Build history of the part. All positions in model axes, mm. Face numbers are marked on the shaded views. A direction names the side the tool comes from. Round coordinates to 2 decimals unless told otherwise and drop trailing zeros. Write each loop counter-clockwise with the first axis right and the second up, starting at its lowest first coordinate (ties: lowest second). Pieces come first, ordered by that corner, then holes. Notation, with made-up numbers: (-35.5, -30) - (7.5, -30) arc R28 ccw to (7.5, -5) - close; hole circle Ø11 at (13, -22). An arc over 180 degrees is marked (long way). One line per question, with ' | ' between items.
from build123d import *

# Parameters (mm, degrees)
F0_W     = 11
F0_H     = 30
F1_DEPTH = 22
F3_DEPTH = 25
F4_R     = 5
F5_DEPTH = 11


with BuildPart() as f1:
    # F0 (on Right) → F1 (new body, symmetric)
    with BuildSketch(Plane.YZ):
        with BuildLine():
            Line((-56, 0), (-30, 0))
            ThreePointArc((-30, 0), (-29.4730143031, 5.5983415304), (-27.9105714739, 11))
            Line((-27.9105714739, 11), (-56, 11))
            Line((-56, 11), (-56, 0))
        make_face()
        with BuildLine():
            ThreePointArc((-27.9105714739, 11), (-29.4730143031, 5.5983415304), (-30, 0))
            Line((-30, 0), (-19, 0))
            ThreePointArc((-19, 0), (-18.1017503893, 5.7729223833), (-15.4919333848, 11))
            Line((-15.4919333848, 11), (-27.9105714739, 11))
        make_face()
        with BuildLine():
            Line((15.4919333848, 11), (27.9105714739, 11))
            ThreePointArc((27.9105714739, 11), (0, 30), (-27.9105714739, 11))
            Line((-27.9105714739, 11), (-15.4919333848, 11))
            ThreePointArc((-15.4919333848, 11), (0, 19), (15.4919333848, 11))
        make_face()
        with BuildLine():
            Line((19, 0), (30, 0))
            ThreePointArc((30, 0), (29.4730143031, 5.5983415304), (27.9105714739, 11))
            Line((27.9105714739, 11), (15.4919333848, 11))
            ThreePointArc((15.4919333848, 11), (18.1017503893, 5.7729223833), (19, 0))
        make_face()
        with BuildLine():
            ThreePointArc((27.9105714739, 11), (29.4730143031, 5.5983415304), (30, 0))
            Line((30, 0), (51, 0))
            Line((51, 0), (51, 11))
            Line((51, 11), (40, 11))
            Line((40, 11), (27.9105714739, 11))
        make_face()
        with Locations((45.5, 26)):
            Rectangle(F0_W, F0_H)
    extrude(amount=F1_DEPTH, both=True)

    # F2 (on face) → F3 (cut)
    with BuildSketch(Plane(origin=(0, 51, 0), x_dir=(-1, 0, 0), z_dir=(0, 1, 0))):
        with BuildLine():
            ThreePointArc((-6.5, 25), (0, 31.5), (6.5, 25))
            Line((6.5, 25), (6.5, 41))
            Line((6.5, 41), (-6.5, 41))
            Line((-6.5, 41), (-6.5, 25))
        make_face()
        with BuildLine():
            Line((-6.5, 25), (6.5, 25))
            ThreePointArc((6.5, 25), (0, 31.5), (-6.5, 25))
        make_face()
        with BuildLine():
            ThreePointArc((-6.5, 25), (0, 18.5), (6.5, 25))
            Line((6.5, 25), (-6.5, 25))
        make_face()
    extrude(amount=-F3_DEPTH, mode=Mode.SUBTRACT)

    # F4 (on face) → F5 (cut, through all)
    with BuildSketch(Plane.XY.offset(11)):
        with Locations((-11, -41.955285737)):
            Circle(F4_R)
        with Locations((11, -41.955285737)):
            Circle(F4_R)
    extrude(amount=-F5_DEPTH, mode=Mode.SUBTRACT)


solid = f1.part
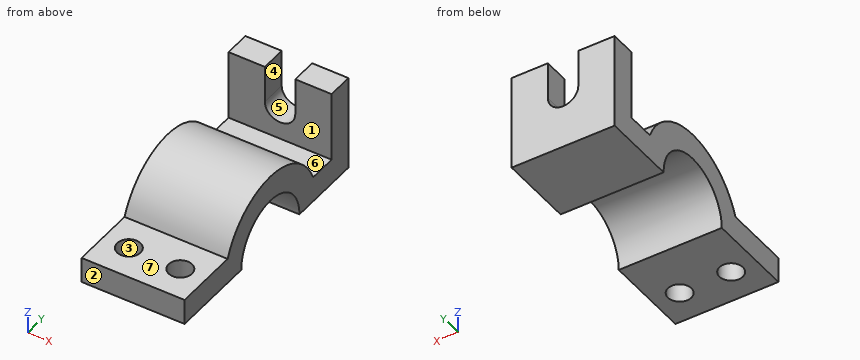
Q1. Saw through at A-A, the plane x = -11. List the corners of the cut face in (y, z).
Found:
outline: (-56, 0) - (-46.96, 0) - (-46.96, 11) - (-56, 11) - close; (-36.96, 0) - (-19, 0) arc R19 cw to (19, 0) - (51, 0) - (51, 41) - (40, 41) - (40, 11) - (27.91, 11) arc R30 ccw to (-27.91, 11) - (-36.96, 11) - close
Q2. Saw through at B-B, the plane z = 13.5. List the corners of the cut face in (x, y), then the cut area to 3 significant figures.
Found:
outline: (-22, -26.79) - (22, -26.79) - (22, -13.37) - (-22, -13.37) - close; (-22, 13.37) - (22, 13.37) - (22, 26.79) - (-22, 26.79) - close; (-22, 40) - (22, 40) - (22, 51) - (-22, 51) - close | area: 1,670 mm^2
Q3. Saw through at D-D, the plane x = 2.5. List the corners of the cut face in (y, z), then the cut area to 3 significant figures.
Found:
outline: (-56, 0) - (-19, 0) arc R19 cw to (19, 0) - (51, 0) - (51, 19) - (40, 19) - (40, 11) - (27.91, 11) arc R30 ccw to (-27.91, 11) - (-56, 11) - close | area: 1,470 mm^2
Q4. Drill centre lines: L1, parallel to Y at x = 11, z = 6; L2, parallel to Y at x = 11, z = 8; L3, parallel to Z at x = 17, y = 33. Where is each one in solid material? Low to high. Write a range as from..to.
Found:
L1: -56..-46.96, -36.96..-18.03, 18.03..51 | L2: -56..-46.96, -36.96..-17.23, 17.23..51 | L3: 0..11
Q5. Saw through at C-C, the plane z = 5.5. List the corners of the cut face in (x, y), then the cut area to 3 significant figures.
Found:
outline: (-22, -56) - (22, -56) - (22, -18.19) - (-22, -18.19) - close; (-22, 18.19) - (22, 18.19) - (22, 51) - (-22, 51) - close; hole circle Ø10 at (-11, -41.96); hole circle Ø10 at (11, -41.96) | area: 2,950 mm^2
Q6. Which spindle directions (+Z, -Z, +X, -X, +Y, -Y) get a long thin tool onto all of the face, cutting with end or side? Do the marked faces 5, 6 and 7. Say none if no direction does.
Found:
face 5: +Z, +Y | face 6: +Z, +X, -X | face 7: +Z, +X, -X, -Y
Q7. Pull direction Y, two halves, no side cores. Call the marked faces 1, 2, 3 and 4: +Y half, -Y half, draft (parallel to the pull), parting line (faces both ways), or undercut.
Found:
face 1: undercut | face 2: -Y half | face 3: undercut | face 4: draft
Q8. Drop flat-ended pins along their axis: pin 1 (3 mm diameter, centred on x = -16.5, z = 13.5, fed in from -Y); pin 2 (9 mm diameter, centred on x = 0, z = 27.5, fed in from -Y); pin 3 (5 mm diameter, centred on x = 8, z = 17.5, fed in from -Y); pin 4 (8 mm diameter, centred on x = -15.5, z = 13, fed in from -Y). Give the stop position or say it passes through.
Found:
pin 1: y = -27.5 | pin 2: y = -19.26 | pin 3: y = -25.98 | pin 4: y = -56
